Answer from the drawing. Dimensions are ordinates in mm from the lowest x, y and z of the part. Round coordinates to 2 decimals unless told otherwise and drop trailing zeros. Loops run counter-clockwise (first coordinate to the right, second up) from the corner with the lowest first, then second, coordinate; pieces in that order, holes last. Notation, with made-up numbers: (0, 79) - (34, 79) arc R26 cw to (34, 98) - close; hole circle Ø2 at (-5.5, 63). An arc over 180 degrees is marked (long way). Answer as CSV lines item,"result".
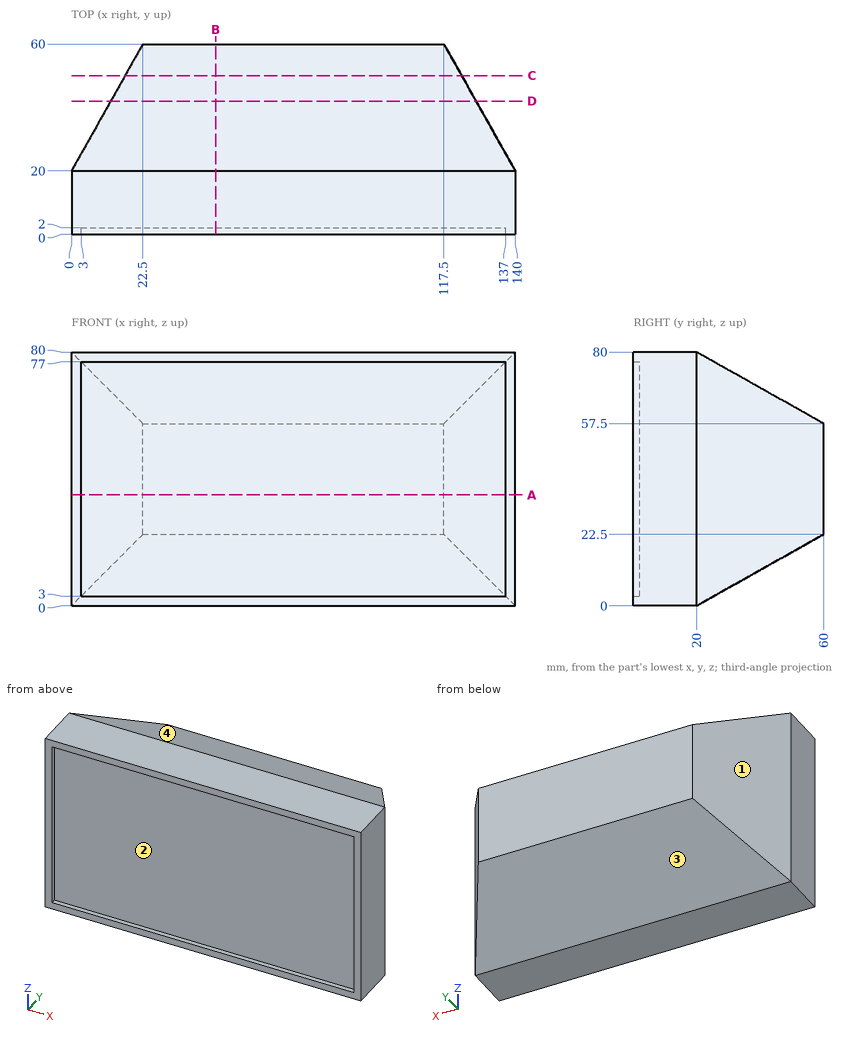
1) A cutting plane is placed at B-B, the plane x = 45.5. Determine the outline of the cut face in (y, z), plus the area to 3 significant figures.
Entries:
outline,"(0, 0) - (20, 0) - (60, 22.5) - (60, 57.5) - (20, 80) - (0, 80) - (0, 77) - (2, 77) - (2, 3) - (0, 3) - close"
area,"3,750 mm^2"
2) A cutting plane is placed at A-A, the plane z = 35. Determine the outline of the cut face in (x, y), plus the area to 3 significant figures.
Entries:
outline,"(0, 0) - (3, 0) - (3, 2) - (137, 2) - (137, 0) - (140, 0) - (140, 20) - (117.5, 60) - (22.5, 60) - (0, 20) - close"
area,"7,230 mm^2"
3) Each of these flat-tipped pins is pushed along its axis until it touches: P1, Ø12, axis at x = 100.5, z = 10.5, coming from the -Y side; P2, Ø3, axis at y = 30.5, z = 31.5, coming from the +X side; P3, Ø8, axis at x = 78.5, z = 64.5, coming from the +Y side. Where does it stop, or does it pass through?
Entries:
P1,"stops at y = 2"
P2,"stops at x = 134.94"
P3,"stops at y = 54.67"
4) Find the intervals of material crossed by line 1 (Y direction, x = 98, z = 36); line 2 (Y direction, x = 103, z = 76.5); line 3 (X direction, y = 25, z = 28), in increasing order.
Entries:
line 1,"y = 2 to 60"
line 2,"y = 2 to 26.22"
line 3,"x = 2.81 to 137.19"
5) A cutting plane is placed at D-D, the plane y = 42. Determine the outline of the cut face in (x, z) (3 decimals).
Entries:
outline,"(12.375, 12.375) - (127.625, 12.375) - (127.625, 67.625) - (12.375, 67.625) - close"
6) The mould has two halves that part along Z. Classify the marked faces 1, 2, 3 and 4: pulls with the +Z half, pulls with the -Z half, needs draft (parallel to the pull), parting line crosses it, or undercut.
Entries:
face 1,"needs draft"
face 2,"undercut"
face 3,"pulls with the -Z half"
face 4,"pulls with the +Z half"
7) A cutting plane is placed at C-C, the plane y = 50. Determine the outline of the cut face in (x, z) (3 decimals), plus the area to 3 significant figures.
Entries:
outline,"(16.875, 16.875) - (123.125, 16.875) - (123.125, 63.125) - (16.875, 63.125) - close"
area,"4,910 mm^2"
